```python
from build123d import *

# Parameters (mm, degrees)
BOSS_EXTRUDE1_DEPTH = 27.5
FILLET1_R           = 3


with BuildPart() as part:
    # Sketch1 → Boss-Extrude1 (new body, symmetric)
    with BuildSketch(Plane.XY):
        with BuildLine():
            Line((-10, 0), (-10, 40))
            Line((-10, 40), (0, 80))
            Line((0, 80), (10, 40))
            Line((10, 40), (10, 0))
            ThreePointArc((10, 0), (0, -10), (-10, 0))
        make_face()
    extrude(amount=BOSS_EXTRUDE1_DEPTH, both=True)

    # Fillet1
    fillet1_edges = [part.edges().sort_by_distance(p)[0] for p in [
        (5, 60, 27.5),
        (-5, 60, 27.5),
        (-10, 20, 27.5),
        (0, -10, 27.5),
        (-10, 20, -27.5),
        (-5, 60, -27.5),
        (5, 60, -27.5),
        (10, 20, -27.5),
        (0, -10, -27.5),
        (10, 20, 27.5),
        (-10, 40, 0),
        (0, 80, 0),
        (10, 40, 0),
    ]]
    fillet(fillet1_edges, radius=FILLET1_R)


solid = part.part
```
Input: part model. Units: mm. Frame: model coordinates. Round coordinates to 2 decimals unless told otherwise and drop trailing zeros. Loops run counter-clockwise (first coordinate to the right, second up) from the corner with the lowest first, then second, coordinate; pieces in that order, holes last.
1) Pin query (flat end, axial travel): pin 1 (2 mm diameter, centred on x = 6.5, z = 8, fed in from -Y); pin 2 (1.5 mm diameter, centred on x = 1.5, z = 17.5, fed in from -Y); pin 3 (4 mm diameter, centred on y = 41.5, z = 17.5, fed in from +X); pin 4 (6 mm diameter, centred on y = 54.5, z = -9, fed in from +X) (3 decimals). Return the tip coordinate at first contact, or that it passes through.
Ans:
pin 1: stops at y = -8.35
pin 2: stops at y = -9.97
pin 3: stops at x = 10
pin 4: stops at x = 7.125
2) Section query A-A on z = 0.5. Return the cut outline in (x, y).
Ans:
outline: (-10, 0) arc R10 ccw to (10, 0) - (10, 39.63) arc R3 ccw to (9.91, 40.36) - (2.91, 68.36) arc R3 ccw to (-2.91, 68.36) - (-9.91, 40.36) arc R3 ccw to (-10, 39.63) - close
3) Material intervals for line 1 (Z direction, x = 1.75, y = 62); line 2 (X direction, y = 60, z = 10); line 3 (X direction, y = 41, z = -5.5), sorted ascending.
Ans:
line 1: z = -27.48 to 27.48
line 2: x = -5 to 5
line 3: x = -9.75 to 9.75
